For this review, use the dimensioned drawing (mm, ordinates from the lowest corner) and the shaded views. Coordinates: 2 decimals unless noted, no trailing zeros. Loops run counter-clockwise (first coordinate to the right, second up) from the corner with the lowest first, then second, coordinate; pieces in that order, holes last. Notation, with made-up numbers: (22, 45) -> (61, 45) arc R24 ccw to (61, 62) -> close; hole circle Ø11 at (-32.5, 81.25). An arc over 180 degrees is marked (long way). Use one line per item in the form item = value. Start each with the question number.
1. Wall thickness on line 1 (X direction, y = 28, z = 8); line 2 (Z direction, x = 90, y = 38); line 3 (Y direction, x = 73.5, z = 16.5): over which ranges is each line inside the solid? List them lowest first. Write a range as from..to.
2. Consider section D-D (y = 67.5). State the section outline as (x, z) points, then the cut area to 3 significant figures.
3. The part is to be moulded in two halves that separate along X. For the marked faces 1, 2 and 3, say which applies: released by +X, released by -X, zero draft, split by the parting line, or undercut.
4. For pin 1 (1.5 mm diameter, centred on x = 62, y = 53, fed in from -Z); pin 2 (12 mm diameter, centred on x = 64.5, y = 53.5, fed in from +Z); pin 3 (4 mm diameter, centred on x = 22, z = 31, fed in from -Y), all flat-tipped, find the tip position at first contact; note any pin that passes through.
5. Consider section C-C (x = 84.5). State the section outline as (y, z) points.
6. Consider section A-A (z = 37.5). State the section outline as (x, y) points.
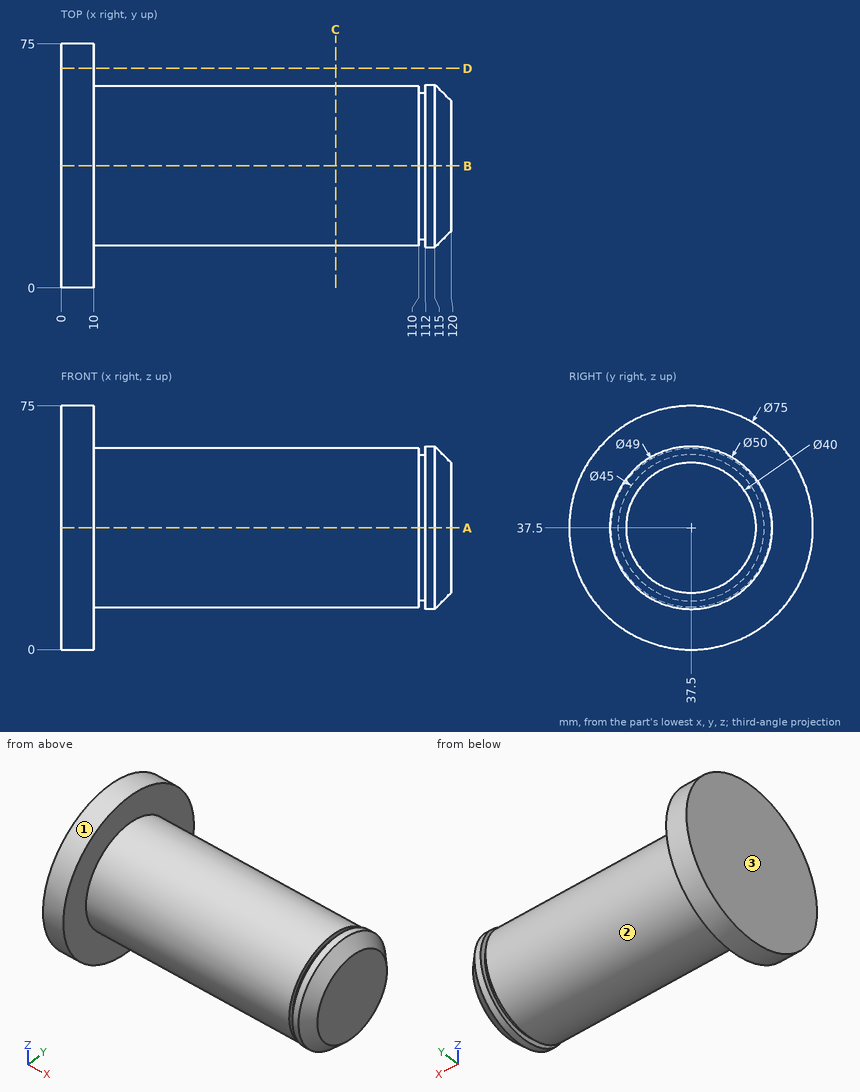
Geometry check:
q1.line_1 = 0..10
q1.line_2 = 13.01..61.99
q1.line_3 = 24.88..50.12
q2.outline = (0, 15) -> (10, 15) -> (10, 60) -> (0, 60) -> close
q2.area = 450 mm²
q3.face_1 = zero draft
q3.face_2 = undercut
q3.face_3 = released by -X
q4.pin_1 = 17.94
q4.pin_2 = 59.87
q4.pin_3 = 13.42
q5.outline = circle Ø49 at (37.5, 37.5)
q6.outline = (0, 0) -> (10, 0) -> (10, 13) -> (110, 13) -> (110, 15) -> (112, 15) -> (112, 12.5) -> (115, 12.5) -> (120, 17.5) -> (120, 57.5) -> (115, 62.5) -> (112, 62.5) -> (112, 60) -> (110, 60) -> (110, 62) -> (10, 62) -> (10, 75) -> (0, 75) -> close
